Geometry: final body of the model. Coordinates: model frame, mm. Face numbers are marked on the shaded views. A direction names the side the tool comes from. Coordinates: 2 decimals unless noted, no trailing zeros. Write each loop counter-clockwise with the first axis right and the second up, starting at its lowest first coordinate (ties: lowest second). Pieces come first, ordered by that corner, then holes. Notation, with made-up numbers: (74.5, 45.25) - (126.5, 45.25) arc R20 ccw to (126.5, 76.25) - close; hole circle Ø2 at (65.5, -11). An arc over 180 degrees is marked (long way). Put each result on its own line as item: value.
```python
from build123d import *

# Parameters (mm, degrees)
F0_R     = 4.2
F1_DEPTH = 10
F5_D     = 8
F5_DEPTH = 15
F6_D     = 8
F6_DEPTH = 15
F7_D     = 6.4
F7_DEPTH = 20


with BuildPart() as f1:
    # F0 (on Top) → F1 (new body)
    with BuildSketch(Plane.XY):
        Polygon((75, -129.903811), (150, 0), (75, 129.903811), (-75, 129.903811), (-150, 0), (-75, -129.903811), align=None)
        with Locations((-95.262794, -55)):
            Circle(F0_R, mode=Mode.SUBTRACT)
        with Locations((0, -110)):
            Circle(F0_R, mode=Mode.SUBTRACT)
        with Locations((95.262794, -55)):
            Circle(F0_R, mode=Mode.SUBTRACT)
        with Locations((-95.262794, 55)):
            Circle(F0_R, mode=Mode.SUBTRACT)
        with Locations((95.262794, 55)):
            Circle(F0_R, mode=Mode.SUBTRACT)
        with Locations((0, 110)):
            Circle(F0_R, mode=Mode.SUBTRACT)
    extrude(amount=F1_DEPTH)

    # F2 (on Front) → F3 (revolve, cut)
    with BuildSketch(Plane.XZ):
        Polygon((-23.5, 2), (-23.5, -10), (0, -10), (0, 18), (-60, 18), (-60, 8), (-22.5, 8), (-22.5, 6.5), (-13, 6.5), (-13, 2), align=None)
    revolve(axis=Axis((0, 0, -2.490325), (0, 0, -1)), mode=Mode.SUBTRACT)

    # F5
    with Locations(Plane.XY.offset(8)):
        with Locations((-9.922068, 51.044614), (39.244898, 34.11507), (49.166966, -16.929544), (9.922068, -51.044614), (-39.244898, -34.11507), (-49.166966, 16.929544)):
            Hole(F5_D / 2, depth=F5_DEPTH)

    # F6
    with Locations(Plane.XY.offset(8)):
        with Locations((-7.498794, 38.577948), (29.660087, 25.78312), (37.15888, -12.794828), (7.498794, -38.577948), (-29.660087, -25.78312), (-37.15888, 12.794828)):
            Hole(F6_D / 2, depth=F6_DEPTH)

    # F7
    with Locations(Plane.XY.offset(8)):
        with Locations((-34.11507, 39.244898), (16.929544, 49.166966), (51.044614, 9.922068), (34.11507, -39.244898), (-16.929544, -49.166966), (-51.044614, -9.922068)):
            Hole(F7_D / 2, depth=F7_DEPTH)


solid = f1.part
```
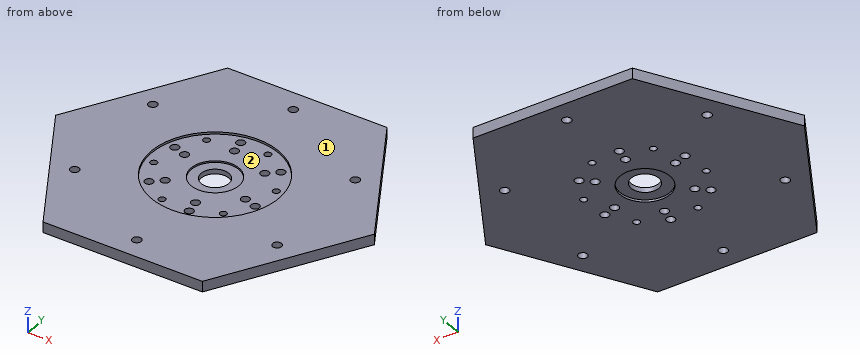
1. Ray query, probe 1 along Y at (x, z) = (-0.5, 1.5); probe 2 along X at (y, z) = (-50, 5); probe 3 along X at (y, z) = (-48, 4.25). Return the intervals inside material, ascending. Write a range as from..to.
Answer below:
probe 1: y = -129.9..-114.17, -105.83..-23.49, 23.49..105.83, 114.17..129.9
probe 2: x = -121.13..-20.02, -13.84..6.06, 13.78..121.13
probe 3: x = -122.29..-19.91, -13.95..7.33, 12.52..122.29
2. Pin query (flat end, axial travel): pin 1 Ø22.5 at (x, y) = (1.5, -9.5) entering from +Z; pin 2 Ø10 at (x, y) = (34.12, -39.24) entering from +Z; pin 3 Ø4 at (y, z) = (32, 5.5) entering from +X. Return the tip coordinate at first contact, or that it passes through.
Answer below:
pin 1: stops at z = 6.5
pin 2: stops at z = 8
pin 3: stops at x = 132.68
3. Set-up query: the marked faces 1 and 2. Return all of +Z, -Z, +X, -X, +Y, -Y with unobstructed straight access to the full face (end or side cutting, diameter ignored); none if empty.
Answer below:
face 1: +Z, +X, -X, +Y, -Y
face 2: +Z
4. Section query B-B (y = 110). Return loops of the section in (x, z).
Answer below:
outline: (-86.49, 0) - (-4.2, 0) - (-4.2, 10) - (-86.49, 10) - close; (4.2, 0) - (86.49, 0) - (86.49, 10) - (4.2, 10) - close
5. Section query D-D (x = 131.5). Return loops of the section in (y, z), then the cut area to 3 significant figures.
Answer below:
outline: (-32.04, 0) - (32.04, 0) - (32.04, 10) - (-32.04, 10) - close
area: 641 mm²
6. Section query A-A (x = 0). Return loops of the section in (y, z).
Answer below:
outline: (-129.9, 0) - (-114.2, 0) - (-114.2, 10) - (-129.9, 10) - close; (-105.8, 0) - (-23.5, 0) - (-23.5, 2) - (-13, 2) - (-13, 6.5) - (-22.5, 6.5) - (-22.5, 8) - (-60, 8) - (-60, 10) - (-105.8, 10) - close; (13, 2) - (23.5, 2) - (23.5, 0) - (105.8, 0) - (105.8, 10) - (60, 10) - (60, 8) - (22.5, 8) - (22.5, 6.5) - (13, 6.5) - close; (114.2, 0) - (129.9, 0) - (129.9, 10) - (114.2, 10) - close
7. Section query C-C (y = -66.5). Return loops of the section in (x, z), then the cut area to 3 significant figures.
Answer below:
outline: (-111.61, 0) - (111.61, 0) - (111.61, 10) - (-111.61, 10) - close
area: 2,230 mm²
